Design review of the part built by this model. Coordinates are the model's own, in mm. Round coordinates to 2 decimals unless told otherwise and drop trailing zeros. Write each loop counter-clockwise with the first axis right and the second up, starting at its lowest first coordinate (ties: lowest second). Pieces come first, ordered by that corner, then holes. Notation, with made-up numbers: (1, 87) - (31, 87) arc R31 cw to (31, 119) - close; hole circle Ø9 at (41.25, 8). An arc over 180 degrees is marked (long way). Use one line per item in the form item = value.
```python
from build123d import *

# Parameters (mm, degrees)
HEXDIESKE_R  = 4.5825
HEXDIE_DEPTH = 0.712


with BuildPart() as part:
    # BodySke → Body (revolve)
    with BuildSketch(Plane.XY, mode=Mode.PRIVATE) as body_sk:
        Polygon((3.56, 0), (4.582, 0), (4.582, 0.712), (3.382, 0.712), (3.382, 1.4596), (3.56, 1.4596), (3.56, 20), (2.805, 20), (2.55, 19.745), (2.55, 0.26008), (2.805, 0.00508), (3.56, 0.00508), align=None)
    revolve(body_sk.sketch.rotate(Axis((0, 0, 0), (0, 1, 0)), 90), axis=Axis((0, 0, 0), (0, 1, 0)))

    # HexDieSke → HexDie (cut)
    with BuildSketch(Plane(origin=(0, 0.712, 0), x_dir=(-1, 0, 0), z_dir=(0, 1, 0))):
        Circle(HEXDIESKE_R)
        Polygon((0, 4.561067127), (3.95, 2.280533563), (3.95, -2.280533563), (0, -4.561067127), (-3.95, -2.280533563), (-3.95, 2.280533563), align=None, mode=Mode.SUBTRACT)
    extrude(amount=-HEXDIE_DEPTH, mode=Mode.SUBTRACT)


solid = part.part
```
Q1. Draft analysis for pull direction Y (two halves, no side actions). For faces 1 (the cylindrical face through (3.302, 1.091, 0.733)), 2 (the flat face through (-3, 0.712, 2)), 3 (the flat face through (-1, 20, -3)), 4 (the cylindrical face through (2.2, 10.9, 2.8)), state which applies: released by +Y, released by -Y, zero draft, split by the parting line, or undercut.
Calculated:
face_1 = undercut
face_2 = undercut
face_3 = released by +Y
face_4 = zero draft
Q2. We need section C-C on y = 13. Write out the cut boundary in (x, z).
Calculated:
outline = circle Ø7.12 at (0, 0); hole circle Ø5.1 at (0, 0)
Q3. We need section A-A on z = 0. Write out the cut boundary in (x, y) (3 decimals).
Calculated:
outline = (-3.95, 0) - (-3.56, 0) - (-3.56, 0.005) - (-2.805, 0.005) - (-2.55, 0.26) - (-2.55, 19.745) - (-2.805, 20) - (-3.56, 20) - (-3.56, 1.46) - (-3.382, 1.46) - (-3.382, 0.712) - (-3.95, 0.712) - close; (2.55, 0.26) - (2.805, 0.005) - (3.56, 0.005) - (3.56, 0) - (3.95, 0) - (3.95, 0.712) - (3.382, 0.712) - (3.382, 1.46) - (3.56, 1.46) - (3.56, 20) - (2.805, 20) - (2.55, 19.745) - close
Q4. To check wall thickness, follow line 1 along X through (y, z) = (10.25, 0); line 2 along X through (y, z) = (9.25, -1); line 3 along Y through (x, z) = (-1.25, -3.5). State the ranges of each line that lie inside material, in increasing order. Write a range as from..to.
Calculated:
line_1 = -3.56..-2.55, 2.55..3.56
line_2 = -3.42..-2.35, 2.35..3.42
line_3 = 0..0.71
Q5. We need section D-D on z = 3.75. Write out the cut boundary in (x, y).
Calculated:
outline = (-1.4, 0) - (1.4, 0) - (1.4, 0.71) - (-1.4, 0.71) - close
Q6. For P1, Ø1.5, axis at y = 9.5, z = -0.5, coming from the +X side; P2, Ø4, axis at x = -1, y = 10, coming from the +Z side; P3, Ø1, axis at y = 5, z = -2, coming from the -X side, all flat-tipped, find the tip position at first contact; note any pin that passes through.
Calculated:
P1 = 3.56
P2 = 3.56
P3 = -3.23
